Read the model definition and answer for the solid it produces. Units are mm, in the model's axes. A direction names the side the tool comes from. Coordinates: 2 decimals unless noted, no trailing zeros. Loops run counter-clockwise (first coordinate to the right, second up) from the corner with the lowest first, then second, coordinate; pieces in that order, holes last.
from build123d import *

# Parameters (mm, degrees)
F1_DEPTH = 25


with BuildPart() as f1:
    # F0 (on Front) → F1 (new body)
    with BuildSketch(Plane.XZ):
        with BuildLine():
            ThreePointArc((-66.516432, -163.946287), (-65.051966, -167.481821), (-61.516432, -168.946287))
            Line((-61.516432, -168.946287), (-18.516432, -168.946287))
            ThreePointArc((-18.516432, -168.946287), (-14.980898, -167.481821), (-13.516432, -163.946287))
            Line((-13.516432, -163.946287), (-13.516432, -162.946287))
            ThreePointArc((-13.516432, -162.946287), (-14.102218, -161.532073), (-15.516432, -160.946287))
            ThreePointArc((-15.516432, -160.946287), (-16.930645, -161.532073), (-17.516432, -162.946287))
            ThreePointArc((-17.516432, -162.946287), (-18.102218, -164.3605), (-19.516432, -164.946287))
            Line((-19.516432, -164.946287), (-24.838233, -164.946287))
            ThreePointArc((-24.838233, -164.946287), (-26.123808, -164.478376), (-26.807848, -163.293583))
            Line((-26.807848, -163.293583), (-35.662202, -113.078046))
            ThreePointArc((-35.662202, -113.078046), (-37.372303, -110.116065), (-40.586241, -108.946287))
            Line((-40.586241, -108.946287), (-61.516432, -108.946287))
            ThreePointArc((-61.516432, -108.946287), (-65.051966, -110.410753), (-66.516432, -113.946287))
            Line((-66.516432, -113.946287), (-66.516432, -163.946287))
        make_face()
        with BuildLine():
            Line((-39.601433, -113.772639), (-30.747079, -163.988176))
            Line((-30.747079, -163.988176), (-30.448126, -164.946287))
            Line((-30.448126, -164.946287), (-61.516432, -164.946287))
            ThreePointArc((-61.516432, -164.946287), (-62.223539, -164.653394), (-62.516432, -163.946287))
            Line((-62.516432, -163.946287), (-62.516432, -113.946287))
            ThreePointArc((-62.516432, -113.946287), (-62.223539, -113.23918), (-61.516432, -112.946287))
            Line((-61.516432, -112.946287), (-40.586241, -112.946287))
            ThreePointArc((-40.586241, -112.946287), (-39.943453, -113.180242), (-39.601433, -113.772639))
        make_face(mode=Mode.SUBTRACT)
    extrude(amount=F1_DEPTH)


solid = f1.part
Item 1: Find the intervals of material crossed by line 1 along Z through (x, y) = (-54, -2.25); line 2 along X through (y, z) = (-20.5, -129.5); line 3 along X through (y, z) = (-12.5, -137.5), in increasing order.
Numbers:
line 1: z = -168.95 to -164.95, -112.95 to -108.95
line 2: x = -66.52 to -62.52, -36.83 to -32.77
line 3: x = -66.52 to -62.52, -35.42 to -31.36
Item 2: A cutting plane is placed at A-A on x = -59. Determine the outline of the cut face in (y, z), then the cut area to 3 significant figures.
Numbers:
outline: (-25, -168.95) - (0, -168.95) - (0, -164.95) - (-25, -164.95) - close; (-25, -112.95) - (0, -112.95) - (0, -108.95) - (-25, -108.95) - close
area: 200 mm2
Item 3: Determine the mould class of faces 1 (the face through (-62.516, -12, -139)), 2 (the face through (-66.516, -12, -139)), 3 (the face through (-65.091, -12.325, -167.443)) for opening direction Z: released by +Z, released by -Z, zero draft, split by the parting line, or undercut.
Numbers:
face 1: undercut
face 2: zero draft
face 3: released by -Z
Item 4: A cutting plane is placed at D-D on z = -135.5. Determine the outline of the cut face in (x, y).
Numbers:
outline: (-66.52, -25) - (-62.52, -25) - (-62.52, 0) - (-66.52, 0) - close; (-35.77, -25) - (-31.71, -25) - (-31.71, 0) - (-35.77, 0) - close
Item 5: Which of the six approach directions +Z, -Z, +X, -X, +Y, -Y give full straight-line access (tool end or side, diameter ignored) to faces 4 (the face through (-46, -12, -164.946)), 5 (the face through (-26.1, -12.3, -164.5)), 6 (the face through (-34, -25, -141))?
Numbers:
face 4: +Y, -Y
face 5: +Z, +Y, -Y
face 6: +Z, -Z, +X, -X, -Y
Item 6: Given pin 1 (2.5 mm diameter, centred on x = -21, y = -8.5, fed in from +Z); pin 2 (3 mm diameter, centred on y = -21.5, z = -121, fed in from +X); pin 3 (7.5 mm diameter, centred on y = -17, z = -138, fed in from +X), each flat-ended and moving along its own axis, determine where each tip first touches the part or whether it passes through.
Numbers:
pin 1: stops at z = -164.95
pin 2: stops at x = -34
pin 3: stops at x = -30.61
Item 7: A cutting plane is placed at B-B on y = -7.5. Determine the outline of the cut face in (x, z), then the cut area to 3 significant figures.
Numbers:
outline: (-66.52, -163.95) arc R5 ccw to (-61.52, -168.95) - (-18.52, -168.95) arc R5 ccw to (-13.52, -163.95) - (-13.52, -162.95) arc R2 ccw to (-15.52, -160.95) arc R2 ccw to (-17.52, -162.95) arc R2 cw to (-19.52, -164.95) - (-24.84, -164.95) arc R2 cw to (-26.81, -163.29) - (-35.66, -113.08) arc R5 ccw to (-40.59, -108.95) - (-61.52, -108.95) arc R5 ccw to (-66.52, -113.95) - close; hole (-62.52, -163.95) arc R1 ccw to (-61.52, -164.95) - (-30.45, -164.95) - (-30.75, -163.99) - (-39.6, -113.77) arc R1 ccw to (-40.59, -112.95) - (-61.52, -112.95) arc R1 ccw to (-62.52, -113.95) - close
area: 750 mm2
Item 8: A cutting plane is placed at C-C on z = -162. Determine the outline of the cut face in (x, y).
Numbers:
outline: (-66.52, -25) - (-62.52, -25) - (-62.52, 0) - (-66.52, 0) - close; (-31.1, -25) - (-27.04, -25) - (-27.04, 0) - (-31.1, 0) - close; (-17.28, -25) - (-13.75, -25) - (-13.75, 0) - (-17.28, 0) - close
